Geometry check sheet. Reference: the model listing, model coordinates, mm. A direction names the side the tool comes from. Coordinates: 2 decimals unless noted, no trailing zeros. Order: outer loops, then holes, each group sorted by start corner. A loop starts at its lowest first (then second) coordinate and runs counter-clockwise, first axis right, second up.
Solid Edge part; units mm, degrees
sketch "Sketch1" plane through (0, 0, 0) normal (0, -1, 0) x (1, 0, 0)
  line L0 (0, 105) -> (15, 105)
  line L1 (15, 90) -> (15, 105)
  line L2 (15, 15) -> (15, 90)
  line L3 (195, 15) -> (15, 15)
  line L4 (195, 51) -> (195, 15)
  line L5 (195, 90) -> (195, 51)
  line L6 (195, 90) -> (195, 105)
  line L7 (195, 105) -> (210, 105)
  line L8 (210, 105) -> (210, 51)
  line L9 (210, 0) -> (210, 51)
  line L10 (0, 0) -> (210, 0)
  line L11 (0, 105) -> (0, 0)
extrude "Protrusion1" add sketch "Sketch1" against normal blind 15
sketch "Sketch2" plane through (202.5, 7.5, 105) normal (0, 0, 1) x (0, -1, 0)
  line L0 (-7.5, -14.98) -> (-7.5, -7.5)
  line L1 (-7.5, -7.5) -> (-0.9713, -7.5)
  line L2 (-0.9713, -7.5) -> (-0.9713, -14.98)
  line L3 (-0.9713, -14.98) -> (-7.5, -14.98)
extrude "ExtrudedProtrusion_9" add sketch "Sketch2" against normal blind 94.0808
sketch "Sketch3" plane through (202.5, 7.5, 105) normal (0, 0, 1) x (0, -1, 0)
  line L0 (-7.5, -180.02) -> (-7.5, -188.3904)
  line L1 (-7.5, -188.3904) -> (-0.9713, -188.3904)
  line L2 (-0.9713, -188.3904) -> (-0.9713, -180.02)
  line L3 (-0.9713, -180.02) -> (-7.5, -180.02)
extrude "Protrusion2" add sketch "Sketch3" against normal up to vertex (105 mm away)
Item 1: Sectioned sample at B-B (y = 12.75). Record the cut outline in (x, z), and give its area (3 significant figures).
Item 2: Tool access check on faces 4 (the face through (191, 8.471, 61)), 5 (the face through (98, 0, 13)), 6 (the face through (22.48, 12, 61)). Record the directions out of +Z, -Z, +X, -X, +Y, -Y that give a thin tool (end or side, any length) a straight path to the whole face; none if there is none.
Item 3: Release check for a two-part mould opening along X. For faces 1 (the face through (15, 4, 59)), 2 (the face through (0, 7, 53)), 3 (the face through (104, 7, 0)) record: pulls with the +X half, pulls with the -X half, needs draft (parallel to the pull), parting line crosses it, or undercut.
Item 4: Thickness scan on line 1 along X through (y, z) = (3, 28); line 2 along X through (y, z) = (11.5, 91.5); line 3 along Z through (x, y) = (57.5, 13). Record the ranges inside material, lowest first.
Item 5: Depth check by flat-ended pin: P1, Ø6, axis at x = 20, z = 45.5, coming from the -Y side; P2, Ø6, axis at x = 126.5, y = 8, coming from the +Z side. Enter the tip coordinate at first touch or a pass-through.
Item 6: Sectioned sample at A-A (z = 66). Record the cut outline in (x, y), and give its area (3 significant figures).
Item 7: Sectioned sample at C-C (x = 161). Record the cut outline in (y, z).
Item 8: Sectioned sample at D-D (y = 2). Record the cut outline in (x, z), and give its area (3 significant figures).
Geometry check:
1. outline: (0, 0) - (210, 0) - (210, 105) - (187.52, 105) - (187.52, 15) - (22.48, 15) - (22.48, 105) - (0, 105) - close
1. area: 7,200 mm2
2. face 4: +Z, -Y
2. face 5: +Z, -Z, +X, -X, -Y
2. face 6: +Z, +Y, -Y
3. face 1: undercut
3. face 2: pulls with the -X half
3. face 3: needs draft
4. line 1: x = 0 to 15, 195 to 210
4. line 2: x = 0 to 22.48, 187.52 to 210
4. line 3: z = 0 to 15
5. P1: stops at y = 8.47
5. P2: stops at z = 15
6. outline: (0, 0) - (15, 0) - (15, 8.47) - (22.48, 8.47) - (22.48, 15) - (0, 15) - close; (187.52, 8.47) - (195, 8.47) - (195, 0) - (210, 0) - (210, 15) - (187.52, 15) - close
6. area: 548 mm2
7. outline: (0, 0) - (15, 0) - (15, 15) - (0, 15) - close
8. outline: (0, 0) - (210, 0) - (210, 105) - (195, 105) - (195, 15) - (15, 15) - (15, 105) - (0, 105) - close
8. area: 5,850 mm2
